Answer from the drawing. Dimensions are ordinates in mm from the lowest x, y and z of the part. A direction names the side the tool comes from. Round coordinates to 2 decimals unless told otherwise and drop trailing zeros. Write each loop counter-clockwise with the first axis right and the second up, starting at its lowest first coordinate (ties: lowest second). Pieces come first, ordered by that corner, then holes. Notation, with made-up numbers: (-22, 31) - (19, 31) arc R28 ccw to (19, 49) - close; hole circle Ø2 at (56.25, 20.5). An arc over 180 degrees is marked (long way). Use a Markdown table: item, result. Add a question column.
1) Each of these flat-tipped pins is pushed along its axis until it touches: P1, Ø5.5, axis at x = 51.78, y = 4.04, coming from the -Z side; P2, Ø8, axis at x = 47, y = 23.5, coming from the -Z side; P3, Ø1, axis at y = 36, z = 8.5, coming from the +X side; P4, Ø1.5, axis at y = 10, z = 10, coming from the -X side. Where does it stop, or does it pass through?
2) Determine the mould class of the marked faces 1, 2, 3 and 4 for opening direction Y: +Y half, -Y half, draft (parallel to the pull), parting line (faces both ways), or undercut.
3) A tool of negligible diameter and unlimited length cuts with its end or side. For the marked faces 5, 6, 7 and 8, from which of +Z, -Z, +X, -X, +Y, -Y can it reach the whole face along a straight path? Write none if from no direction.
4) A cutting plane is placed at B-B (x = 27). Give the vertices of the cut face in (y, z).
5) A cutting plane is placed at A-A (z = 9.25). Give the vertices of the cut face in (x, y) (1 decimal), then the cut area to 3 significant figures.
6) A cutting plane is placed at D-D (y = 41). Give the vertices of the cut face in (x, z).
7) Find the intervals of material crossed by probe 1 along X at (y, z) = (36, 8); probe 2 along X at (y, z) = (20, 10.75); probe 3 along Y at (x, z) = (50, 7.75) (1 decimal), in increasing order. Write a range as from..to.
8) A cutting plane is placed at C-C (y = 29). Give the vertices of the cut face in (x, z), then the cut area to 3 significant figures.
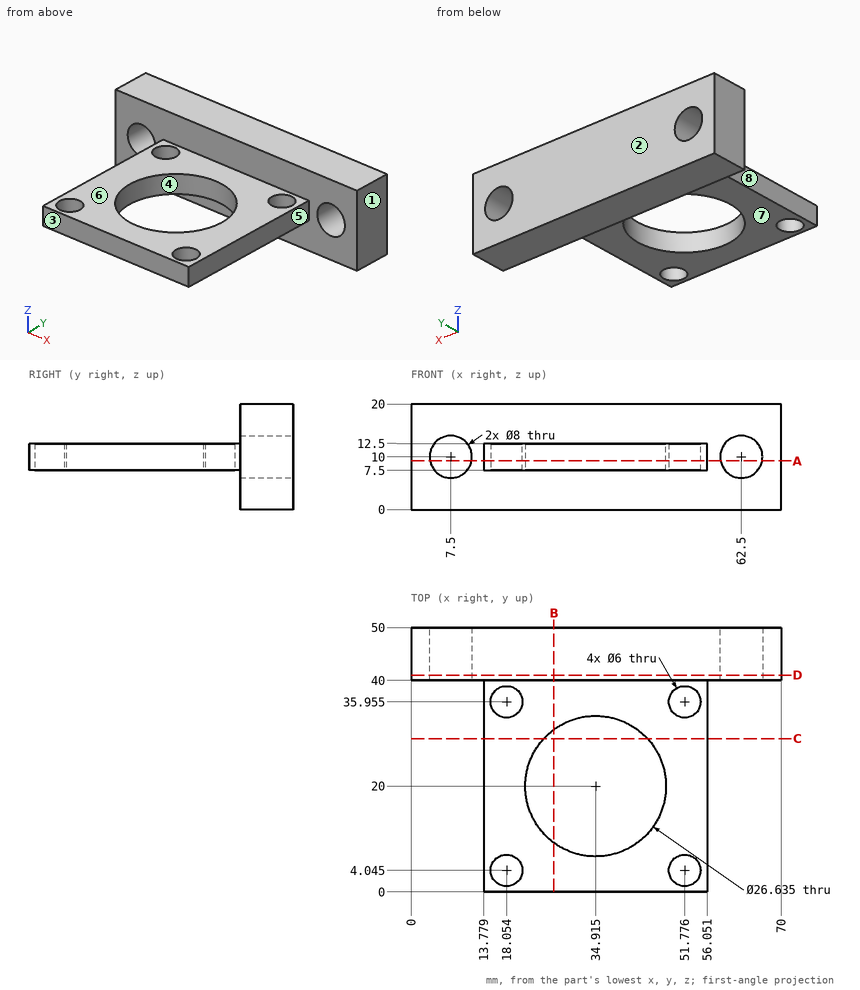
Entries:
| question | item | result |
|---|---|---|
| 1 | P1 | passes through |
| 1 | P2 | stops at z = 7.5 |
| 1 | P3 | stops at x = 56.05 |
| 1 | P4 | stops at x = 13.78 |
| 2 | face 1 | draft |
| 2 | face 2 | +Y half |
| 2 | face 3 | -Y half |
| 2 | face 4 | undercut |
| 3 | face 5 | +Z, -Z, +X, -Y |
| 3 | face 6 | +Z, +X, -X, -Y |
| 3 | face 7 | -Z, +X, -X, -Y |
| 3 | face 8 | +Z, -Z, -X, -Y |
| 4 | outline | (0, 7.5) - (9.29, 7.5) - (9.29, 12.5) - (0, 12.5) - close; (30.71, 7.5) - (40, 7.5) - (40, 0) - (50, 0) - (50, 20) - (40, 20) - (40, 12.5) - (30.71, 12.5) - close |
| 5 | outline | (0, 40) - (3.6, 40) - (3.6, 50) - (0, 50) - close; (11.4, 40) - (13.8, 40) - (13.8, 0) - (56.1, 0) - (56.1, 40) - (58.6, 40) - (58.6, 50) - (11.4, 50) - close; (66.4, 40) - (70, 40) - (70, 50) - (66.4, 50) - close; hole circle Ø6 at (18.1, 4); hole circle Ø6 at (18.1, 36); hole circle Ø26.6 at (34.9, 20); hole circle Ø6 at (51.8, 4); hole circle Ø6 at (51.8, 36) |
| 5 | area | 1,560 mm² |
| 6 | outline | (0, 0) - (70, 0) - (70, 20) - (0, 20) - close; hole circle Ø8 at (7.5, 10); hole circle Ø8 at (62.5, 10) |
| 7 | probe 1 | x = 13.78..15.05, 21.05..48.78, 54.78..56.05 |
| 7 | probe 2 | x = 13.78..21.6, 48.23..56.05 |
| 7 | probe 3 | y = 0..1.6, 6.5..33.5, 38.4..50 |
| 8 | outline | (13.78, 7.5) - (25.1, 7.5) - (25.1, 12.5) - (13.78, 12.5) - close; (44.73, 7.5) - (56.05, 7.5) - (56.05, 12.5) - (44.73, 12.5) - close |
| 8 | area | 113 mm² |
